Input: part model. Units: mm. Frame: model coordinates. Coordinates: 2 decimals unless noted, no trailing zeros. Order: outer loops, then holes, each group sorted by start corner. A loop starts at its lowest first (then second) coordinate and runs counter-clockwise, first axis right, second up. Notation, with made-up numbers: M 56,2 L 94,2 A24 cw 94,13 Z; hole C -22.5,48 d3. An arc over 180 degrees is marked long. One line per item, written item: value.
Autodesk Inventor part; units mm, degrees
ref_plane "YZ Plane" through (0, 0, 0) normal (1, 0, 0) x (0, 1, 0)
ref_plane "XZ Plane" through (0, 0, 0) normal (0, 1, 0) x (-1, 0, 0)
ref_plane "XY Plane" through (0, 0, 0) normal (0, 0, 1) x (1, 0, 0)
sketch "Skizze1" plane through (0, 0, 0) normal (1, 0, 0) x (0, 1, 0)
  line L0 (10, 30) -> (-10, 30)
  line L1 (-10, 30) -> (-10, 10)
  line L2 (-10, 10) -> (-30.5, 10)
  line L3 (-30.5, 10) -> (-30.5, -10)
  line L4 (-30.5, -10) -> (-30.5, -10)
  line L5 (-30.5, -10) -> (-10.5, -45)
  line L6 (10, 0) -> (10, 30)
  arc A0 (28, -37) -> (27.8513, -15.001) centre (28, -26) ccw
  arc A1 (10, 0) -> (27.8513, -15.001) centre (26, 0.918) ccw
  arc A2 (-10.5, -45) -> (9.7132, -46.2044) centre (0, -39) ccw
  arc A3 (28, -37) -> (9.7132, -46.2044) centre (28, -59.7678) ccw
  point P0 (0, 0)
  point P1 (-30.5, 0)
  point P2 (0, 30)
  dimension "d0" = 20
  dimension "d1" = 20
  dimension "d3" = 40
  dimension "d6" = 0
  dimension "d41" = 20
  dimension "d43" = 22
  dimension "d45" = 18
  dimension "d56" = 16
  dimension "d60" = 45
  dimension "d61" = 39
  dimension "d62" = 10
  dimension "d63" = 18
  dimension "d67" = 26
  dimension "d68" = 0.918
extrude "Extrusion1" add sketch "Skizze1" along normal mid plane 4
fillet "Rundung1" radius 2 5 edges at (0, 10, 30) (0, -10, 30) (0, -10, 10) (0, -30.5, 10) (0, -30.5, -10)
sketch "Skizze2" plane through (2, 0, 0) normal (1, 0, 0) x (0, 0, -1)
  circle A0 centre (-20, 0) radius 2.5
  circle A1 centre (0, 0) radius 2.5
  circle A2 centre (0, -20.5) radius 2.5
  circle A3 centre (39, 0) radius 7.9
  line L0 (-8, -30.5) -> (9.4689, -30.5)
  line L1 (-30, 8) -> (-30, -8)
  line L2 (0, 10) -> (-28, 10)
  circle A4 centre (26, 28) radius 2.5
  arc A5 (37, 28) -> (15.001, 27.8513) centre (26, 28) ccw
  point P0 (0, 0)
  point P1 (0.7344, -30.5)
  dimension "d10" = 5
  dimension "d11" = 5
  dimension "d12" = 5
  dimension "d13" = 10
  dimension "d14" = 20
  dimension "d15" = 10
  dimension "d16" = 15.8
  dimension "d58" = 0
  dimension "d64" = 5
  dimension "d69" = 39
extrude "Extrusion2" cut sketch "Skizze2" against normal through all
properties part number "KettenBlech_Oben_Hinten"
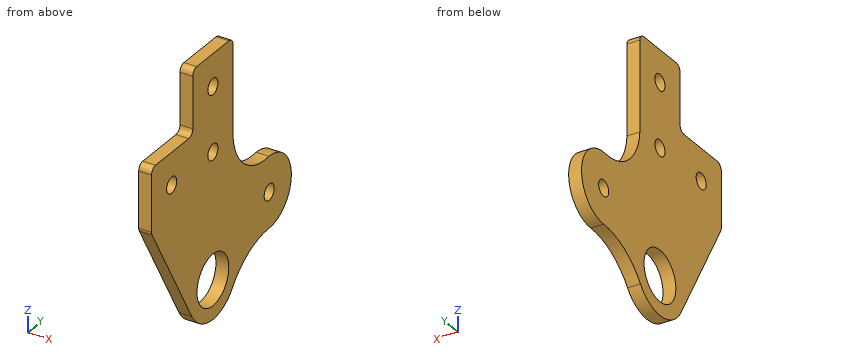
(1) Ray query, line 1 (Y direction, x = 0.3, z = 0); line 2 (Z direction, x = 0.7, y = 0.5); line 3 (Y direction, x = 0.95, z = 7). Return the intervals inside material, ascending. Write a range as from..to.
Data:
line 1: y = -30.5..-23, -18..-2.5, 2.5..10
line 2: z = -51.08..-46.88, -31.12..-2.45, 2.45..17.55, 22.45..30
line 3: y = -30.5..10
(2) First-contact query: pin 1 (1.2 mm diameter, centred on x = 0, z = 18, fed in from -Y); pin 2 (4 mm diameter, centred on y = -20.5, z = 0, fed in from +X); pin 3 (1 mm diameter, centred on x = 0, y = -12.5, fed in from +Z); pin 4 (1.5 mm diameter, centred on x = 1.5, z = -38, fed in from -Y). Flat tips, straight axial feed; report the tip coordinate or a pass-through.
Data:
pin 1: stops at y = -10
pin 2: passes through
pin 3: stops at z = 10
pin 4: stops at y = -14.93
(3) Cut plane C-C on z = -32. Output: boundary loops of the cut face in (x, y).
Data:
outline: M -2,-17.93 L 2,-17.93 L 2,-3.66 L -2,-3.66 Z; M -2,3.66 L 2,3.66 L 2,37.22 L -2,37.22 Z
(4) Cut plane B-B on y = -20.5. Output: boundary loops of the cut face in (x, z), plus the area to 3 significant figures.
Data:
outline: M -2,-27.5 L 2,-27.5 L 2,-2.5 L -2,-2.5 Z; M -2,2.5 L 2,2.5 L 2,10 L -2,10 Z
area: 130 mm2
(5) Cut plane A-A on y = 0. Output: boundary loops of the cut face in (x, z), plus the area to 3 significant figures.
Data:
outline: M -2,-51.09 L 2,-51.09 L 2,-46.9 L -2,-46.9 Z; M -2,-31.1 L 2,-31.1 L 2,-2.5 L -2,-2.5 Z; M -2,2.5 L 2,2.5 L 2,17.5 L -2,17.5 Z; M -2,22.5 L 2,22.5 L 2,30 L -2,30 Z
area: 221 mm2
(6) Cut plane D-D on x = -0.45. Output: boundary loops of the cut face in (y, z), plus the area to 3 significant figures.
Data:
outline: M -30.5,-9.47 A2 ccw -30.24,-10.46 L -10.5,-45 A12.09 ccw 9.71,-46.2 A22.77 cw 28,-37 A11 ccw long 27.85,-15 A16.03 cw 10,0 L 10,28 A2 ccw 8,30 L -8,30 A2 ccw -10,28 L -10,12 A2 cw -12,10 L -28.5,10 A2 ccw -30.5,8 Z; hole C -20.5,0 d5; hole C 0,-39 d15.8; hole C 0,0 d5; hole C 0,20 d5; hole C 28,-26 d5
area: 2,780 mm2
